Input: part model. Units: mm. Frame: model coordinates. A direction names the side the tool comes from. Give positions to 0.01 mm unless a question says otherwise; leave off trailing zeros. Loops run counter-clockwise (first coordinate to the right, second up) from the corner with the lowest first, then second, coordinate; pieces in that order, holes last. Notation, with made-up numbers: M -22.5,83 L 2.5,83 A19 ccw 2.5,115 Z; hole C -35.75,24.25 d1. An arc over 180 degrees is marked long. One line per item, written item: value. Start each with the question number.
(1) Pull-direction query (X, two-part tool) for faces 5 (the flat face through (30, -0.1, -59.8)), 6 (the flat face through (26, -9.5, -40)), 7 (the cylindrical face through (19.535, -15.01, -44.776)); classes: released by +X, released by -X, zero draft, split by the parting line, or undercut.
(2) Ray query, line 1 along Z through (x, y) = (-27, 0); line 2 along X through (y, z) = (13.5, -25); line 3 along X through (y, z) = (1, -49). Return the intervals inside material, ascending. Write a range as from..to.
(3) Section C-C on y = 11. Output: boundary loops of the cut face in (x, z).
(4) Section D-D on y = -3. State how many separate pieces and enclosed holes the cut face has, plus the area to 3 significant figures.
(5) Pin query (flat end, axial travel): P1, Ø3.5, axis at x = -8.5, y = -15.5, coming from the -Z side; P2, Ø1.1, axis at y = -0.5, z = -63, coming from the +X side; P3, Ø7.5, axis at y = 0, z = -17, coming from the -X side; P4, Ø1.2, axis at x = 0.5, z = -45.5, coming from the +Y side. Return the tip coordinate at first contact, or that it passes through.
(6) Section A-A on x = -6. Output: boundary loops of the cut face in (y, z), plus the area to 3 significant figures.
(7) Section B-B on z = -11. Output: boundary loops of the cut face in (x, y), plus the area to 3 significant figures.
(8) Access query for faces 1 (the cylindrical face through (22.99, -3.459, -34.155)), 2 (the flat face through (26, -12, -44)), 3 (the flat face through (0, -15, -45.929)), 4 (the flat face through (0, 16, -49.85)). Directions: +Z, -Z, +X, -X, +Y, -Y. A direction counts if a zero-diameter tool reaches every point of the face in a straight line with its end or side. Return the directions, or none.
Autodesk Inventor part; units mm, degrees
ref_plane "clip1_to_dummy_XY" through (0, 0, -17) normal (1, 0, 0) x (0, 0, -1)
ref_plane "clip1_to_dummy_YZ" through (0, 0, -17) normal (0, 0, -1) x (0, 1, 0)
ref_plane "clip1_to_dummy_ZX" through (0, 0, -17) normal (0, 1, 0) x (1, 0, 0)
sketch "Sketch_1" plane through (0, 0, 0) normal (0, 0, 1) x (1, 0, 0)
  line L0 (-30, 17) -> (-30, -17)
  line L1 (-30, -17) -> (30, -17)
  line L2 (30, -17) -> (30, 17)
  line L3 (30, 17) -> (-30, 17)
extrude "Extrusion1" add sketch "Sketch_1" against normal blind 79
sketch "Sketch_3" plane through (0, 0, 0) normal (0, 0, 1) x (1, 0, 0)
  line L0 (-22, 12) -> (-22, -17)
  line L1 (-22, -17) -> (22, -17)
  line L2 (22, -17) -> (22, 12)
  line L3 (22, 12) -> (-22, 12)
extrude "Extrusion2" cut sketch "Sketch_3" along normal mid plane 158
sketch "Sketch_6" plane through (0, 0, -31.85) normal (0, 0, 1) x (1, 0, 0)
  line L0 (-13.2, 18.02) -> (-12.289, 14.62)
  line L1 (-12.289, 14.62) -> (12.289, 14.62)
  line L2 (12.289, 14.62) -> (13.2, 18.02)
  line L3 (13.2, 18.02) -> (-13.2, 18.02)
extrude "Extrusion3" cut sketch "Sketch_6" against normal blind 18
sketch "Sketch_4" plane through (0, 0, 0) normal (0, 1, 0) x (-1, 0, 0)
  line L0 (60, 60) -> (-60, 60)
  line L1 (-60, 60) -> (-60, -120)
  line L2 (-60, -120) -> (60, -120)
  line L3 (60, -120) -> (60, 60)
  line L4 (30, 0) -> (22, 0)
  line L5 (22, 0) -> (22, -27.2)
  line L6 (22, -27.2) -> (-22, -27.2)
  line L7 (-22, -27.2) -> (-22, 0)
  line L8 (-22, 0) -> (-30, 0)
  line L9 (-30, 0) -> (-30, -79)
  line L10 (-30, -79) -> (-22, -79)
  line L11 (-22, -79) -> (-22, -55.2)
  line L12 (-22, -55.2) -> (22, -55.2)
  line L13 (22, -55.2) -> (22, -79)
  line L14 (22, -79) -> (30, -79)
  line L15 (30, -79) -> (30, 0)
extrude "Extrusion4" cut sketch "Sketch_4" along normal mid plane 158
sketch "Sketch_2" plane through (0, 0, 0) normal (1, 0, 0) x (0, 1, 0)
  line L0 (45, 45) -> (-45, 45)
  line L1 (-45, 45) -> (-45, -90)
  line L2 (-45, -90) -> (45, -90)
  line L3 (45, -90) -> (45, 45)
  arc A0 (17, -17) -> (-17, -17) centre (0, -17) ccw
  line L4 (-17, -17) -> (-17, -62)
  arc A1 (-17, -62) -> (17, -62) centre (0, -62) ccw
  line L5 (17, -62) -> (17, -17)
extrude "Extrusion5" cut sketch "Sketch_2" along normal mid plane 60
sketch "Sketch_5" plane through (-25.8, 0, 0) normal (1, 0, 0) x (0, 0, -1)
  arc A0 (49.4116, 12.1565) -> (62, -17.5) centre (62, 0) ccw
  line L0 (62, -17.5) -> (62, -56)
  line L1 (62, -56) -> (89.4, -56)
  line L2 (89.4, -56) -> (89.4, 47)
  line L3 (89.4, 47) -> (63.4892, 47)
  line L4 (63.4892, 47) -> (49.4116, 12.1565)
  circle A1 centre (62, 0) radius 4.25
extrude "Extrusion6" cut sketch "Sketch_5" against normal blind 15
sketch "Sketch_8" plane through (-25.8, 0, 0) normal (1, 0, 0) x (0, 0, -1)
  circle A0 centre (62, 0) radius 1.8889
extrude "Extrusion7" cut sketch "Sketch_8" against normal blind 15
sketch "Sketch_11" plane through (0, 0, 0) normal (1, 0, 0) x (0, 1, 0)
  circle A0 centre (0, -17) radius 4.25
extrude "Extrusion8" cut sketch "Sketch_11" along normal mid plane 60
sketch "Sketch_24" plane through (-26, 0, 0) normal (1, 0, 0) x (0, 0, -1)
  line L0 (-3.4, -51) -> (17, -51)
  line L1 (17, -51) -> (17, -17.5)
  arc A0 (17, -17.5) -> (29.5884, 12.1565) centre (17, 0) ccw
  line L2 (29.5884, 12.1565) -> (21.5712, 32)
  line L3 (21.5712, 32) -> (-3.4, 32)
  line L4 (-3.4, 32) -> (-3.4, -51)
extrude "Extrusion9" cut sketch "Sketch_24" along normal blind 52
sketch "Sketch_7" plane through (25.8, 0, 0) normal (1, 0, 0) x (0, 0, -1)
  arc A0 (49.4116, 12.1565) -> (55.6364, -16.302) centre (62, 0) ccw
  arc A1 (62, -25.6174) -> (55.6364, -16.302) centre (52, -25.6174) ccw
  line L0 (62, -25.6174) -> (62, -56)
  line L1 (62, -56) -> (89.4, -56)
  line L2 (89.4, -56) -> (89.4, 47)
  line L3 (89.4, 47) -> (63.4892, 47)
  line L4 (63.4892, 47) -> (49.4116, 12.1565)
  circle A2 centre (62, 0) radius 4.25
extrude "Extrusion10" cut sketch "Sketch_7" along normal blind 15
sketch "Sketch_9" plane through (25.8, 0, 0) normal (1, 0, 0) x (0, 0, -1)
  circle A0 centre (62, 0) radius 1.8889
extrude "Extrusion11" cut sketch "Sketch_9" along normal blind 15
sketch "Sketch_10" plane through (0, 0, -39.5) normal (0, 0, 1) x (1, 0, 0)
  line L0 (-30, -8) -> (-30, -11)
  line L1 (-30, -11) -> (-28.4, -11)
  line L2 (-28.4, -11) -> (-28.4, -17)
  line L3 (-28.4, -17) -> (-22, -17)
  line L4 (-22, -17) -> (-22, -8)
  line L5 (-22, -8) -> (-30, -8)
  circle A0 centre (-24, -12) radius 1.55
extrude "Extrusion12" cut sketch "Sketch_10" along normal mid plane 9
sketch "Sketch_13" plane through (0, 0, -39.5) normal (0, 0, 1) x (1, 0, 0)
  line L0 (22, -8) -> (22, -17)
  line L1 (22, -17) -> (28.4, -17)
  line L2 (28.4, -17) -> (28.4, -11)
  line L3 (28.4, -11) -> (30, -11)
  line L4 (30, -11) -> (30, -8)
  line L5 (30, -8) -> (22, -8)
  circle A0 centre (24, -12) radius 1.55
extrude "Extrusion13" cut sketch "Sketch_13" along normal mid plane 9
sketch "Sketch_14" plane through (0, 0, 0) normal (0, 1, 0) x (-1, 0, 0)
  line L0 (-28.6667, -66.25) -> (-30, -62)
  line L1 (-30, -62) -> (-30, -66.25)
  line L2 (-30, -66.25) -> (-28.6667, -66.25)
extrude "Extrusion14" cut sketch "Sketch_14" along normal mid plane 8.5
sketch "Sketch_18" plane through (0, 0, 0) normal (0, 1, 0) x (-1, 0, 0)
  line L0 (30, -62) -> (28.6667, -66.25)
  line L1 (28.6667, -66.25) -> (30, -66.25)
  line L2 (30, -66.25) -> (30, -62)
extrude "Extrusion15" cut sketch "Sketch_18" along normal mid plane 8.5
sketch "Sketch_25" plane through (0, 0, -39.5) normal (0, 0, 1) x (1, 0, 0)
  line L0 (-27.4, -9.5) -> (-27.4, -13.4)
  arc A0 (-27.4, -13.4) -> (-23.8, -17) centre (-23.8, -13.4) ccw
  line L1 (-23.8, -17) -> (23.8, -17)
  arc A1 (23.8, -17) -> (27.4, -13.4) centre (23.8, -13.4) ccw
  line L2 (27.4, -13.4) -> (27.4, -9.5)
  line L3 (27.4, -9.5) -> (25.55, -9.5)
  line L4 (25.55, -9.5) -> (25.55, -12)
  arc A2 (22.45, -12) -> (25.55, -12) centre (24, -12) ccw
  line L5 (22.45, -12) -> (-22.45, -12)
  arc A3 (-25.55, -12) -> (-22.45, -12) centre (-24, -12) ccw
  line L6 (-25.55, -12) -> (-25.55, -9.5)
  line L7 (-25.55, -9.5) -> (-27.4, -9.5)
extrude "Extrusion16" add sketch "Sketch_25" along normal mid plane 8.1818
sketch "Sketch_27" plane through (0, 0, -39.5) normal (0, 0, 1) x (1, 0, 0)
  arc A0 (-21.2467, -16.6281) -> (-21.1445, -17) centre (-21.1445, -16.8) ccw
  line L0 (-21.1445, -17) -> (21.1445, -17)
  arc A1 (21.1445, -17) -> (21.2467, -16.6281) centre (21.1445, -16.8) ccw
  arc A2 (18.6673, -12.75) -> (21.2467, -16.6281) centre (24, -12) ccw
  line L1 (18.6673, -12.75) -> (-18.6673, -12.75)
  arc A3 (-21.2467, -16.6281) -> (-18.6673, -12.75) centre (-24, -12) ccw
extrude "Extrusion17" add sketch "Sketch_27" along normal mid plane 12.8571
ref_plane "clip1_to_dummy_XY" through (0, 0, -17) normal (1, 0, 0) x (0, 0, -1)
ref_plane "clip1_to_dummy_YZ" through (0, 0, -17) normal (0, 0, -1) x (0, 1, 0)
ref_plane "clip1_to_dummy_ZX" through (0, 0, -17) normal (0, 1, 0) x (1, 0, 0)
ref_plane "clip_back_to_clip_front_XY" through (0, 0, -62) normal (1, 0, 0) x (0, 0, -1)
ref_plane "clip_back_to_clip_front_YZ" through (0, 0, -62) normal (0, 0, -1) x (0, 1, 0)
ref_plane "clip_back_to_clip_front_ZX" through (0, 0, -62) normal (0, 1, 0) x (1, 0, 0)
ref_plane "clip_end_to_fitting_free_left_XY" through (-25.8, 0, -917) normal (1, 0, 0) x (0, 0, -1)
ref_plane "clip_end_to_fitting_free_left_YZ" through (-25.8, 0, -917) normal (0, 0, -1) x (0, 1, 0)
ref_plane "clip_end_to_fitting_free_left_ZX" through (-25.8, 0, -917) normal (0, 1, 0) x (1, 0, 0)
ref_plane "clip_end_to_fitting_free_right_XY" through (25.8, 0, -917) normal (1, 0, 0) x (0, 0, -1)
ref_plane "clip_end_to_fitting_free_right_YZ" through (25.8, 0, -917) normal (0, 0, -1) x (0, 1, 0)
ref_plane "clip_end_to_fitting_free_right_ZX" through (25.8, 0, -917) normal (0, 1, 0) x (1, 0, 0)
ref_plane "clip_front_to_clip_back_XY" through (0, 0, -17) normal (1, 0, 0) x (0, 0, -1)
ref_plane "clip_front_to_clip_back_YZ" through (0, 0, -17) normal (0, 0, -1) x (0, 1, 0)
ref_plane "clip_front_to_clip_back_ZX" through (0, 0, -17) normal (0, 1, 0) x (1, 0, 0)
ref_plane "clip_front_to_fitting_fixed_left_XY" through (-26, 0, -17) normal (1, 0, 0) x (0, 0, -1)
ref_plane "clip_front_to_fitting_fixed_left_YZ" through (-26, 0, -17) normal (0, 0, -1) x (0, 1, 0)
ref_plane "clip_front_to_fitting_fixed_left_ZX" through (-26, 0, -17) normal (0, 1, 0) x (1, 0, 0)
ref_plane "clip_front_to_fitting_fixed_right_XY" through (26, 0, -17) normal (1, 0, 0) x (0, 0, -1)
ref_plane "clip_front_to_fitting_fixed_right_YZ" through (26, 0, -17) normal (0, 0, -1) x (0, 1, 0)
ref_plane "clip_front_to_fitting_fixed_right_ZX" through (26, 0, -17) normal (0, 1, 0) x (1, 0, 0)
ref_plane "clip_front_to_fitting_right_XY" through (0, 0, -17) normal (1, 0, 0) x (0, 0, -1)
ref_plane "clip_front_to_fitting_right_YZ" through (0, 0, -17) normal (0, 0, -1) x (0, 1, 0)
ref_plane "clip_front_to_fitting_right_ZX" through (0, 0, -17) normal (0, 1, 0) x (1, 0, 0)
ref_plane "clip_to_flap_XY" through (-24, -12, -39.5) normal (0, 0, 1) x (1, 0, 0)
ref_plane "clip_to_flap_YZ" through (-24, -12, -39.5) normal (1, 0, 0) x (0, 1, 0)
ref_plane "clip_to_flap_ZX" through (-24, -12, -39.5) normal (0, 1, 0) x (0, 0, 1)
ref_plane "to_center_XY" through (0, 44.6514, -39.5) normal (1, 0, 0) x (0, 0, -1)
ref_plane "to_center_YZ" through (0, 44.6514, -39.5) normal (0, 0, -1) x (0, 1, 0)
ref_plane "to_center_ZX" through (0, 44.6514, -39.5) normal (0, 1, 0) x (1, 0, 0)
ref_plane "to_clip1_XY" through (0, 0, -17) normal (0, 0, 1) x (1, 0, 0)
ref_plane "to_clip1_YZ" through (0, 0, -17) normal (1, 0, 0) x (0, 1, 0)
ref_plane "to_clip1_ZX" through (0, 0, -17) normal (0, 1, 0) x (0, 0, 1)
ref_plane "to_clip5_XY" through (0, 0, -917) normal (0, 0, 1) x (1, 0, 0)
ref_plane "to_clip5_YZ" through (0, 0, -917) normal (1, 0, 0) x (0, 1, 0)
ref_plane "to_clip5_ZX" through (0, 0, -917) normal (0, 1, 0) x (0, 0, 1)
properties part number "MHPUS306-50-25-Aclip"
Output values:
1. face 5: released by +X
1. face 6: zero draft
1. face 7: undercut
2. line 1: z = -66.25..-63.89, -60.11..-57.75, -44.5..-21.25, -12.75..0
2. line 2: x = -30..-26, 26..30
2. line 3: x = -25.8..-22, 22..25.8
3. outline: M -30,-48.39 L -25.8,-48.39 L -25.8,-74.96 L -22,-74.96 L -22,-30.61 L -26,-30.61 L -26,-4.04 L -30,-4.04 Z; M 22,-74.96 L 25.8,-74.96 L 25.8,-48.39 L 30,-48.39 L 30,-4.04 L 26,-4.04 L 26,-30.61 L 22,-30.61 Z
4. separate pieces: 4
4. enclosed holes: 0
4. area: 698 mm²
5. P1: stops at z = -45.93
5. P2: stops at x = 25.8
5. P3: passes through
5. P4: stops at y = 14.62
6. outline: M -17,-45.93 L -12.75,-45.93 L -12.75,-43.59 L -12,-43.59 L -12,-35.41 L -12.75,-35.41 L -12.75,-33.07 L -17,-33.07 Z; M 12,-55.2 L 17,-55.2 L 17,-49.85 L 14.62,-49.85 L 14.62,-31.85 L 17,-31.85 L 17,-27.63 L 12.16,-29.59 A17.5 cw 12,-29.74 Z
6. area: 151 mm²
7. outline: M -30,-15.91 L -26,-15.91 L -26,15.91 L -30,15.91 Z; M 26,-15.91 L 30,-15.91 L 30,15.91 L 26,15.91 Z
7. area: 254 mm²
8. face 1: +Z
8. face 2: none
8. face 3: -Z, -Y
8. face 4: +Y
